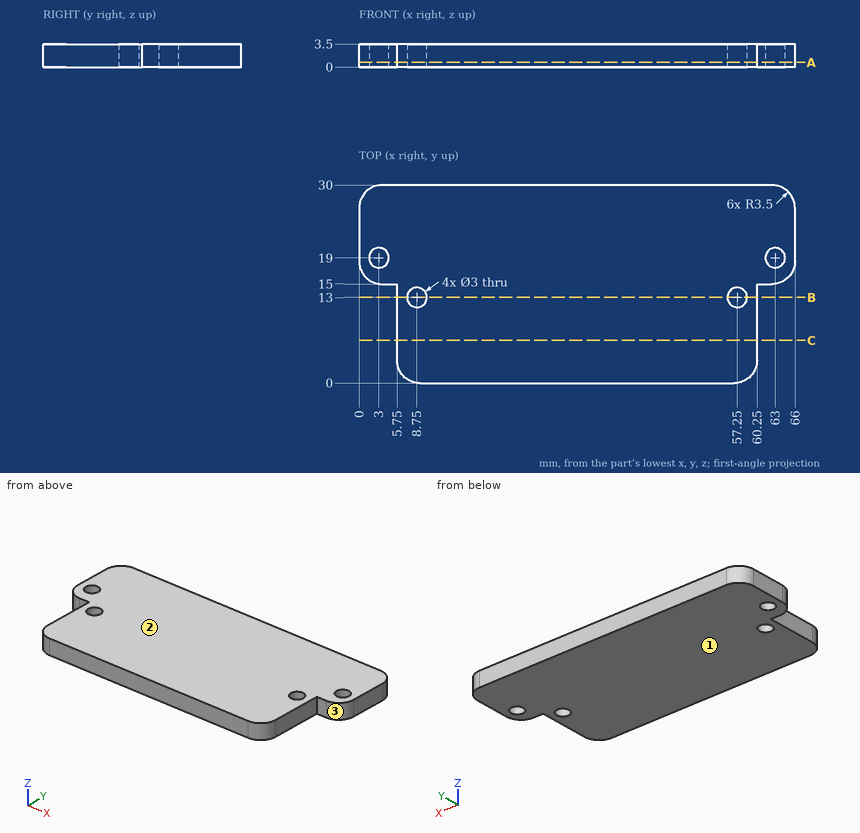
Answer from the drawing. Dimensions are ordinates in mm from the lowest x, y and z of the part. Coordinates: 2 decimals unless noted, no trailing zeros. Loops run counter-clockwise (first coordinate to the right, second up) from the corner with the lowest first, then second, coordinate; pieces in that order, holes last. Notation, with made-up numbers: (-32.5, 20) -> (9.5, 20) arc R37 cw to (9.5, 57) -> close; hole circle Ø2 at (70.25, 3.25). An arc over 180 degrees is marked (long way). Answer in a Markdown table with one row per item.
Item 1: Straight lines are drawn through the part: line 1 along Y through (x, z) = (8.75, 1.3); line 2 along Y through (x, z) = (3, 1.35); line 3 along X through (y, z) = (5.75, 3.1). For each, find the intervals that lie inside material, in ascending order. Write a range as [from, to].
Returned:
| item | result |
|---|---|
| line 1 | y = [0.04, 11.5], [14.5, 30] |
| line 2 | y = [15.04, 17.5], [20.5, 29.96] |
| line 3 | x = [5.75, 60.25] |
Item 2: A cutting plane is placed at B-B on y = 13. Determine the outline of the cut face in (x, z).
Returned:
| item | result |
|---|---|
| outline | (5.75, 0) -> (7.25, 0) -> (7.25, 3.5) -> (5.75, 3.5) -> close; (10.25, 0) -> (55.75, 0) -> (55.75, 3.5) -> (10.25, 3.5) -> close; (58.75, 0) -> (60.25, 0) -> (60.25, 3.5) -> (58.75, 3.5) -> close |
Item 3: A cutting plane is placed at A-A on z = 0.7. Determine the outline of the cut face in (x, y), plus the area to 3 significant figures.
Returned:
| item | result |
|---|---|
| outline | (0, 18.5) arc R3.5 ccw to (3.5, 15) -> (5.75, 15) -> (5.75, 3.5) arc R3.5 ccw to (9.25, 0) -> (56.75, 0) arc R3.5 ccw to (60.25, 3.5) -> (60.25, 15) -> (62.5, 15) arc R3.5 ccw to (66, 18.5) -> (66, 26.5) arc R3.5 ccw to (62.5, 30) -> (3.5, 30) arc R3.5 ccw to (0, 26.5) -> close; hole circle Ø3 at (3, 19); hole circle Ø3 at (8.75, 13); hole circle Ø3 at (57.25, 13); hole circle Ø3 at (63, 19) |
| area | 1,760 mm^2 |
Item 4: Each of these flat-tipped pins is pushed along its axis until it touches: P1, Ø1.8, axis at x = 3, y = 19, coming from the +Z side (3 decimals); P2, Ø1.5, axis at x = 7.5, z = 3, coming from the -Y side; P3, Ø1.1, axis at x = 62, z = 1.5, coming from the -Y side. Where does it stop, or does it pass through?
Returned:
| item | result |
|---|---|
| P1 | passes through |
| P2 | stops at y = 0.15 |
| P3 | stops at y = 15 |
Item 5: A cutting plane is placed at C-C on y = 6.5. Determine the outline of the cut face in (x, z).
Returned:
| item | result |
|---|---|
| outline | (5.75, 0) -> (60.25, 0) -> (60.25, 3.5) -> (5.75, 3.5) -> close |
Item 6: For a pull along Z with two mould halves and no side action, classify the marked faces 1, 2 and 3 as released by +Z, released by -Z, zero draft, split by the parting line, or undercut.
Returned:
| item | result |
|---|---|
| face 1 | released by -Z |
| face 2 | released by +Z |
| face 3 | zero draft |
